Autodesk Inventor part; units mm, degrees
ref_plane "YZ Plane" through (0, 0, 0) normal (1, 0, 0) x (0, 1, 0)
ref_plane "XZ Plane" through (0, 0, 0) normal (0, 1, 0) x (-1, 0, 0)
ref_plane "XY Plane" through (0, 0, 0) normal (0, 0, 1) x (1, 0, 0)
sketch "Sketch1" plane through (0, 0, 0) normal (0, 1, 0) x (-1, 0, 0)
  line L0 (75, 0) -> (75, -100)
  line L1 (75, -100) -> (-75, -100)
  line L2 (-75, -100) -> (-75, 100)
  line L3 (-75, 100) -> (75, 100)
  line L4 (75, 100) -> (75, 0)
  line L5 (75, 100) -> (75, 70)
  line L6 (75, -100) -> (75, -70)
  line L7 (-75, -100) -> (-75, -70)
  line L8 (-75, 100) -> (-75, 70)
  line L9 (75, 70) -> (75, 50)
  line L10 (-75, 70) -> (-75, 50)
  line L11 (-75, -70) -> (-75, -50)
  line L12 (75, -70) -> (75, -50)
  line L13 (75, -70) -> (72.5, -70)
  line L14 (72.5, -70) -> (72.5, -50)
  line L15 (72.5, -50) -> (75, -50)
  line L16 (-75, -70) -> (-72.5, -70)
  line L17 (-72.5, -70) -> (-72.5, -50)
  line L18 (-72.5, -50) -> (-75, -50)
  line L19 (75, 70) -> (72.5, 70)
  line L20 (72.5, 70) -> (72.5, 50)
  line L21 (72.5, 50) -> (75, 50)
  line L22 (-75, 70) -> (-72.5, 70)
  line L23 (-72.5, 70) -> (-72.5, 50)
  line L24 (-72.5, 50) -> (-75, 50)
  line L25 (-75, -100) -> (-75, -97)
  line L26 (-75, -100) -> (-72, -100)
  circle A0 centre (-69.4679, -94.4422) radius 3
  circle A1 centre (69.3699, -94.4422) radius 3
  circle A2 centre (69.3699, 94.4217) radius 3
  circle A3 centre (-69.4679, 94.4217) radius 3
  line L27 (75, -50) -> (75, -35)
  line L28 (75, 50) -> (75, 35)
  line L29 (75, -35) -> (75, -25)
  line L30 (75, 35) -> (75, 25)
  line L31 (75, -25) -> (75, -21)
  line L32 (75, -21) -> (75, -17)
  line L33 (75, -17) -> (75, -13)
  line L34 (75, -13) -> (75, -9)
  line L35 (75, -9) -> (75, -5)
  line L36 (75, -5) -> (75, -1)
  line L37 (75, -1) -> (75, 3)
  line L38 (75, 3) -> (75, 7)
  line L39 (75, 7) -> (75, 11)
  line L40 (75, 11) -> (75, 15)
  line L41 (75, 15) -> (75, 19)
  line L42 (75, 19) -> (75, 23)
  circle A4 centre (60, 30) radius 5
  circle A5 centre (-60, 30) radius 5
  circle A6 centre (0, 30) radius 5
  line L43 (0, -35) -> (0, -30)
  circle A7 centre (0, -30) radius 5
  circle A8 centre (-60, -30) radius 5
  circle A9 centre (60, -30) radius 5
  circle A10 centre (0, -15) radius 2
  circle A11 centre (20, -15) radius 2
  circle A12 centre (44, -15) radius 2
  circle A13 centre (-21, -15) radius 2
  circle A14 centre (-43, -15) radius 2
  circle A15 centre (44, -7) radius 2
  circle A16 centre (20, -7) radius 2
  circle A17 centre (0, -7) radius 2
  circle A18 centre (-21, -7) radius 2
  circle A19 centre (-43, -7) radius 2
  circle A20 centre (44, 1) radius 2
  circle A21 centre (20, 1) radius 2
  circle A22 centre (0, 1) radius 2
  circle A23 centre (-21, 1) radius 2
  circle A24 centre (-43, 1) radius 2
  circle A25 centre (44, 9) radius 2
  circle A26 centre (20, 9) radius 2
  circle A27 centre (0, 9) radius 2
  circle A28 centre (-21, 9) radius 2
  circle A29 centre (-43, 9) radius 2
  circle A30 centre (44, 17) radius 2
  circle A31 centre (20, 17) radius 2
  circle A32 centre (0, 17) radius 2
  circle A33 centre (-21, 17) radius 2
  circle A34 centre (-43, 17) radius 2
  point P0 (0, 0)
  dimension "d3" = 150
  dimension "d4" = 200
  dimension "d6" = 30
  dimension "d7" = 30
  dimension "d8" = 30
  dimension "d9" = 30
  dimension "d10" = 20
  dimension "d11" = 20
  dimension "d12" = 20
  dimension "d13" = 20
  dimension "d14" = 2.5
  dimension "d15" = 2.5
  dimension "d16" = 2.5
  dimension "d17" = 2.5
  dimension "d20" = 6
  dimension "d23" = 6
  dimension "d26" = 6
  dimension "d28" = 6
  dimension "d30" = 15
  dimension "d31" = 15
  dimension "d32" = 10
  dimension "d33" = 10
  dimension "d34" = 4
  dimension "d35" = 4
  dimension "d47" = 10
  dimension "d49" = 10
  dimension "d50" = 10
  dimension "d51" = 5
  dimension "d52" = 10
  dimension "d55" = 10
  dimension "d56" = 10
  dimension "d58" = 4
  dimension "d59" = 4
  dimension "d60" = 4
  dimension "d61" = 4
  dimension "d62" = 4
  dimension "d63" = 4
  dimension "d64" = 4
  dimension "d65" = 4
  dimension "d66" = 4
  dimension "d67" = 4
  dimension "d68" = 4
  dimension "d69" = 4
  dimension "d70" = 4
  dimension "d71" = 4
  dimension "d72" = 4
  dimension "d73" = 4
  dimension "d74" = 4
  dimension "d75" = 4
  dimension "d76" = 4
  dimension "d77" = 4
  dimension "d78" = 4
  dimension "d79" = 4
  dimension "d80" = 4
  dimension "d81" = 4
  dimension "d82" = 4
extrude "Extrusion1" add sketch "Sketch1" along normal blind 5 contours L0 L15 L14 L13 L1 L2 L16 L17 L18 L24 L23 L22 L3 L4 L19 L20 L21
extrude "Extrusion2" add sketch "Sketch1" along normal blind 30 contours L2 L18 L17 L16
extrude "Extrusion3" add sketch "Sketch1" along normal blind 30 contours L0 L13 L14 L15
extrude "Extrusion4" add sketch "Sketch1" along normal blind 30 contours L21 L20 L19 L4
extrude "Extrusion5" add sketch "Sketch1" along normal blind 30 contours L22 L23 L24 L2
sketch "Sketch2" plane through (0, 5, 0) normal (0, 1, 0) x (1, 0, 0)
  point P0 (0, 0)
sketch "Sketch3" plane through (0, 5, 0) normal (0, 1, 0) x (1, 0, 0)
  point P0 (0, 0)
  point P1 (-75, 100)
properties part number "Base"
Could you check a few things on this model? Use its own coordinates, in mm. A direction names the side the tool comes from. Round coordinates to 2 decimals unless told otherwise and drop trailing zeros. Write each loop counter-clockwise with the first axis right and the second up, starting at its lowest first coordinate (ties: lowest second). Pieces come first, ordered by that corner, then holes.
(1) For pin 1 (2 mm diameter, centred on x = -73.5, y = 23.5, fed in from +Z); pin 2 (5 mm diameter, centred on x = 21, z = 1, fed in from +Y); pin 3 (3 mm diameter, centred on x = -73.5, y = 19, fed in from -Z), each with a flat end and sliding along its axis, tell me the tip position at first contact or that it passes through.
Findings below:
pin 1: stops at z = 70
pin 2: stops at y = 5
pin 3: stops at z = -70
(2) Suppose I cut it at D-D on x = -57.5. Write out the boundary of the cut face in (y, z), and give its area (3 significant figures).
Findings below:
outline: (0, -100) - (5, -100) - (5, -34.33) - (0, -34.33) - close; (0, -25.67) - (5, -25.67) - (5, 25.67) - (0, 25.67) - close; (0, 34.33) - (5, 34.33) - (5, 100) - (0, 100) - close
area: 913 mm2
(3) Which directions (+Z, -Z, +X, -X, +Y, -Y) give clear straight access to the entire face, cutting with the end or side of a thin tool? Please do faces 1 (the face through (-16, 0, 1)), 2 (the face through (-72.5, 17, -60)).
Findings below:
face 1: +Z, -Z, +X, -X, -Y
face 2: +Z, -Z, +Y
(4) If I drill on probe 1 along Z at (x, y) = (43, 1.55); probe 2 along Z at (x, y) = (-60, 1.3); probe 3 along X at (y, z) = (13.25, 59.5), over which ranges is the centre line in solid material (lowest first)?
Findings below:
probe 1: z = -100 to -17, -13 to -9, -5 to -1, 3 to 7, 11 to 15, 19 to 100
probe 2: z = -100 to -35, -25 to 25, 35 to 100
probe 3: x = -75 to -72.5, 72.5 to 75
(5) Suppose I cut it at A-A on x = 60. Write out the boundary of the cut face in (y, z).
Findings below:
outline: (0, -100) - (5, -100) - (5, -35) - (0, -35) - close; (0, -25) - (5, -25) - (5, 25) - (0, 25) - close; (0, 35) - (5, 35) - (5, 100) - (0, 100) - close
(6) Thinking about a two-plate mould opening in Z: for faces 3 (the face through (-1, 2, -100)), 4 (the face through (72.5, 17, 60)), 5 (the face through (66.606, 2.465, -95.343)), which applies, +Z half, -Z half, draft (parallel to the pull), parting line (faces both ways), or undercut?
Findings below:
face 3: -Z half
face 4: draft
face 5: undercut
(7) Suppose I cut it at C-C on y = 24.5. Write out the boundary of the cut face in (x, z), and give its area (3 significant figures).
Findings below:
outline: (-75, -70) - (-72.5, -70) - (-72.5, -50) - (-75, -50) - close; (-75, 50) - (-72.5, 50) - (-72.5, 70) - (-75, 70) - close; (72.5, -70) - (75, -70) - (75, -50) - (72.5, -50) - close; (72.5, 50) - (75, 50) - (75, 70) - (72.5, 70) - close
area: 200 mm2
(8) Suppose I cut it at B-B on z = -30. Write out the boundary of the cut face in (x, y).
Findings below:
outline: (-75, 0) - (-65, 0) - (-65, 5) - (-75, 5) - close; (-55, 0) - (-5, 0) - (-5, 5) - (-55, 5) - close; (5, 0) - (55, 0) - (55, 5) - (5, 5) - close; (65, 0) - (75, 0) - (75, 5) - (65, 5) - close
